from build123d import *

# Parameters (mm, degrees)
SKETCH1_W           = 150
SKETCH1_H           = 34
BOSS_EXTRUDE1_DEPTH = 35
CUT_EXTRUDE1_DEPTH  = 160
SKETCH7_R           = 3.75
CUT_EXTRUDE9_DEPTH  = 160
CUT_EXTRUDE11_DEPTH = 158.737123088
SKETCH8_W           = 0.25
SKETCH8_H           = 34
CUT_EXTRUDE12_DEPTH = 158.737123088
SKETCH9_R           = 4
CUT_EXTRUDE13_DEPTH = 5


with BuildPart() as part:
    # Sketch1 → Boss-Extrude1 (new body)
    with BuildSketch(Plane.XY):
        with Locations((75, 17)):
            Rectangle(SKETCH1_W, SKETCH1_H)
    extrude(amount=BOSS_EXTRUDE1_DEPTH)

    # Sketch2 → Cut-Extrude1 (cut)
    with BuildSketch(Plane(origin=(150, 0, 0), x_dir=(0, 0, -1), z_dir=(1, 0, 0))):
        Polygon((-35, 17), (-35, 19), (-10, 19), (-10, 15), (-35, 15), align=None)
    extrude(amount=-CUT_EXTRUDE1_DEPTH, mode=Mode.SUBTRACT)

    # Sketch7 → Cut-Extrude9 (cut)
    with BuildSketch(Plane(origin=(150, 0, 0), x_dir=(0, 0, -1), z_dir=(1, 0, 0))):
        with Locations((-17.5, 26.5)):
            Circle(SKETCH7_R)
        with Locations((-17.5, 7.5)):
            Circle(SKETCH7_R)
    extrude(amount=-CUT_EXTRUDE9_DEPTH, mode=Mode.SUBTRACT)

    # Sketch3 → Cut-Extrude11 (cut, through all)
    with BuildSketch(Plane(origin=(150, 0, 0), x_dir=(0, 0, -1), z_dir=(1, 0, 0))):
        Polygon((-33.7, 19.75), (-35, 20.5), (-35, 19), align=None)
        Polygon((-33.7, 21.25), (-35, 22), (-35, 20.5), align=None)
        Polygon((-33.7, 22.75), (-35, 23.5), (-35, 22), align=None)
        Polygon((-33.7, 24.25), (-35, 25), (-35, 23.5), align=None)
        Polygon((-33.7, 25.75), (-35, 26.5), (-35, 25), align=None)
        Polygon((-33.7, 27.25), (-35, 28), (-35, 26.5), align=None)
        Polygon((-33.7, 28.75), (-35, 29.5), (-35, 28), align=None)
        Polygon((-33.7, 30.25), (-35, 31), (-35, 29.5), align=None)
        Polygon((-35, 34.75), (-35, 34), (-33.7, 34.75), align=None)
        Polygon((-35, 34), (-35, 32.5), (-33.7, 33.25), align=None)
        Polygon((-33.7, 31.75), (-35, 32.5), (-35, 31), align=None)
    cut_extrude11 = extrude(amount=-CUT_EXTRUDE11_DEPTH, mode=Mode.SUBTRACT)

    # Mirror1: Cut-Extrude11 across plane
    add(cut_extrude11.mirror(Plane.ZX.offset(17)), mode=Mode.SUBTRACT)

    # Sketch8 → Cut-Extrude12 (cut, through all)
    with BuildSketch(Plane(origin=(150, 0, 0), x_dir=(0, 0, -1), z_dir=(1, 0, 0))):
        with Locations((-34.875, 17)):
            Rectangle(SKETCH8_W, SKETCH8_H)
    extrude(amount=-CUT_EXTRUDE12_DEPTH, mode=Mode.SUBTRACT)

    # Sketch9 → Cut-Extrude13 (cut)
    with BuildSketch(Plane(origin=(0, 0, 0), x_dir=(-1, 0, 0), z_dir=(0, 0, -1))):
        with Locations((-50, 17)):
            Circle(SKETCH9_R)
        with Locations((-100, 17)):
            Circle(SKETCH9_R)
    extrude(amount=-CUT_EXTRUDE13_DEPTH, mode=Mode.SUBTRACT)


solid = part.part
Input: part model. Units: mm. Frame: model coordinates. A direction names the side the tool comes from. Give positions to 0.01 mm unless a question says otherwise; leave off trailing zeros. Order: outer loops, then holes, each group sorted by start corner. A loop starts at its lowest first (then second) coordinate and runs counter-clockwise, first axis right, second up. Notation, with made-up numbers: M -4,69 L 3,69 A21 cw 3,84 Z; hole C 31.25,4 d3. An arc over 180 degrees is marked long. Answer as a JSON object with one key per item and string values.
1. Cut plane A-A, the plane z = 17.5. Output: boundary loops of the cut face in (x, y).
Result sheet:
{"outline": "M 0,0 L 150,0 L 150,3.75 L 0,3.75 Z; M 0,11.25 L 150,11.25 L 150,15 L 0,15 Z; M 0,19 L 150,19 L 150,22.75 L 0,22.75 Z; M 0,30.25 L 150,30.25 L 150,34 L 0,34 Z"}
2. Cut plane D-D, the plane x = 50. State how many separate pieces and enclosed holes the cut face has, and give its area (3 significant figures).
Result sheet:
{"separate pieces": "1", "enclosed holes": "2", "area": "941 mm²"}
3. First-contact query: P1, Ø3, axis at x = 52, y = 17, coming from the +Z side; P2, Ø4, axis at x = 51.5, y = 16.5, coming from the -Z side. Flat tips, straight axial feed; report the tip coordinate or a pass-through.
Result sheet:
{"P1": "z = 10", "P2": "z = 5"}
4. Cut plane C-C, the plane y = 17. Output: boundary loops of the cut face in (x, z).
Result sheet:
{"outline": "M 0,0 L 46,0 L 46,5 L 54,5 L 54,0 L 96,0 L 96,5 L 104,5 L 104,0 L 150,0 L 150,10 L 0,10 Z"}
5. Ray query, line 1 (Y direction, x = 9, z = 20.5); line 2 (Y direction, x = 102.5, z = 17.5); line 3 (Y direction, x = 100, z = 1). Return the intervals inside material, ascending. Write a range as [from, to].
Result sheet:
{"line 1": "[0, 5.25], [9.75, 15], [19, 24.25], [28.75, 34]", "line 2": "[0, 3.75], [11.25, 15], [19, 22.75], [30.25, 34]", "line 3": "[0, 13], [21, 34]"}
6. Pull-direction query (Z, two-part tool) for faces 4 (the cylindrical face through (76.05, 22.84, 18.31)), 5 (the flat face through (76, 19, 23)), 6 (the flat face through (50, 17, 5)); classes: +Z half, -Z half, draft (parallel to the pull), parting line (faces both ways), or undercut.
Result sheet:
{"face 4": "undercut", "face 5": "draft", "face 6": "-Z half"}
7. Cut plane B-B, the plane z = 25.5. Output: boundary loops of the cut face in (x, y), and give its area (3 significant figures).
Result sheet:
{"outline": "M 0,0 L 150,0 L 150,15 L 0,15 Z; M 0,19 L 150,19 L 150,34 L 0,34 Z", "area": "4,500 mm²"}
8. Reachability of faces 1 (the flat face through (74, 17, 0)), 2 (the cylindrical face through (52.95, 19.7, 2.46)), 3 (the flat face through (76, 17, 10)) from +Z, -Z, +X, -X, +Y, -Y: full face, straight path, thin tool, end or side. Return the list, or none.
Result sheet:
{"face 1": "-Z, +X, -X, +Y, -Y", "face 2": "-Z", "face 3": "+Z, +X, -X"}
